Input: part model. Units: mm. Frame: model coordinates. A direction names the side the tool comes from. Give positions to 0.01 mm unless a question says otherwise; leave off trailing zeros. Loops run counter-clockwise (first coordinate to the right, second up) from the corner with the lowest first, then second, coordinate; pieces in that order, holes last.
from build123d import *

# Parameters (mm, degrees)
SKETCH1_W           = 40
SKETCH1_H           = 40
SKETCH1_R           = 3.175
BOSS_EXTRUDE1_DEPTH = 9
SKETCH2_W           = 40
SKETCH2_H           = 6
BOSS_EXTRUDE2_DEPTH = 35
FILLET1_R           = 3.175
SKETCH3_R           = 3.175
CUT_EXTRUDE1_DEPTH  = 63.737548565


with BuildPart() as part:
    # Sketch1 → Boss-Extrude1 (new body)
    with BuildSketch(Plane.XY):
        Rectangle(SKETCH1_W, SKETCH1_H)
        with Locations((9, 0)):
            Circle(SKETCH1_R, mode=Mode.SUBTRACT)
        with Locations((-9, 0)):
            Circle(SKETCH1_R, mode=Mode.SUBTRACT)
    extrude(amount=BOSS_EXTRUDE1_DEPTH)

    # Sketch2 → Boss-Extrude2 (add)
    with BuildSketch(Plane.XY.offset(9)):
        with Locations((0, 17)):
            Rectangle(SKETCH2_W, SKETCH2_H)
        with Locations((0, -17)):
            Rectangle(SKETCH2_W, SKETCH2_H)
    extrude(amount=BOSS_EXTRUDE2_DEPTH)

    # Fillet1
    fillet1_edges = [part.edges().sort_by_distance(p)[0] for p in [
        (0, -14, 9),
        (0, 14, 9),
    ]]
    fillet(fillet1_edges, radius=FILLET1_R)

    # Sketch3 → Cut-Extrude1 (cut, through all)
    with BuildSketch(Plane(origin=(0, 20, 0), x_dir=(1, 0, 0), z_dir=(0, 1, 0))):
        with BuildLine():
            Line((-20, -44), (1e-09, -44))
            add(Edge.make_bspline(
                [(-20, -26), (-20, -44), (0, -44)],
                knots=[3.141592654, 3.141592654, 3.141592654, 4.71238898, 4.71238898, 4.71238898], degree=2, weights=[1, 0.707106781, 1]))
            Line((-20, -26), (-20, -44))
        make_face()
        with BuildLine():
            Line((1e-09, -44), (20, -44))
            Line((20, -44), (20, -26))
            add(Edge.make_bspline(
                [(0, -44), (20, -44), (20, -26)],
                knots=[4.71238898, 4.71238898, 4.71238898, 6.283185307, 6.283185307, 6.283185307], degree=2, weights=[1, 0.707106781, 1]))
        make_face()
        with Locations(Location((0, -26, 0), (0, 0, 270))):
            Circle(SKETCH3_R)
    extrude(amount=-CUT_EXTRUDE1_DEPTH, mode=Mode.SUBTRACT)


solid = part.part
(1) Cut plane D-D (y = -9). Return the cut outline in (x, z).
Values follow:
outline: (-20, 0) - (20, 0) - (20, 9) - (-20, 9) - close
(2) Cut plane A-A (y = 0). Return the cut outline in (x, z) (3 decimals), and give its area (3 significant figures).
Values follow:
outline: (-20, 0) - (-12.175, 0) - (-12.175, 9) - (-20, 9) - close; (-5.825, 0) - (5.825, 0) - (5.825, 9) - (-5.825, 9) - close; (12.175, 0) - (20, 0) - (20, 9) - (12.175, 9) - close
area: 246 mm2
(3) Mould query, pull axis Y, two halves, no side actions, for faces 1 (the flat face through (0, 20, 22)), 2 (the cylindrical face through (0.14, 17.04, 22.83)), 3 (the cylindrical face through (12.03, 0.95, 4.44)), 4 (the flat face through (4, -14, 28)). Classes: +Y half, -Y half, draft (parallel to the pull), parting line (faces both ways), or undercut.
Values follow:
face 1: +Y half
face 2: draft
face 3: undercut
face 4: undercut
(4) Reachability of faces 5 (the flat face through (4, 14, 28)), 6 (the flat face through (0, -20, 22)) from +Z, -Z, +X, -X, +Y, -Y: full face, straight path, thin tool, end or side. Return the list, or none.
Values follow:
face 5: +Z, +X, -X
face 6: +Z, -Z, +X, -X, -Y
(5) Ray query, probe 1 along Y at (x, z) = (2, 40.5); probe 2 along X at (y, z) = (-16.95, 26) (3 decimals). Return the intervals inside material, ascending.
Values follow:
probe 1: y = -20 to -14, 14 to 20
probe 2: x = -20 to -3.175, 3.175 to 20
(6) Pin query (flat end, axial travel): pin 1 Ø6 at (x, y) = (5.5, 7) entering from +Z. Return the tip coordinate at first contact, or that it passes through.
Values follow:
pin 1: stops at z = 9
(7) Cut plane B-B (z = 13.5). Return the cut outline in (x, y), and give its area (3 significant figures).
Values follow:
outline: (-20, -20) - (20, -20) - (20, -14) - (-20, -14) - close; (-20, 14) - (20, 14) - (20, 20) - (-20, 20) - close
area: 480 mm2
(8) Cut plane C-C (z = 8). Return the cut outline in (x, y) (3 decimals), and give its area (3 significant figures).
Values follow:
outline: (-20, -20) - (20, -20) - (20, 20) - (-20, 20) - close; hole circle Ø6.35 at (-9, 0); hole circle Ø6.35 at (9, 0)
area: 1,540 mm2
